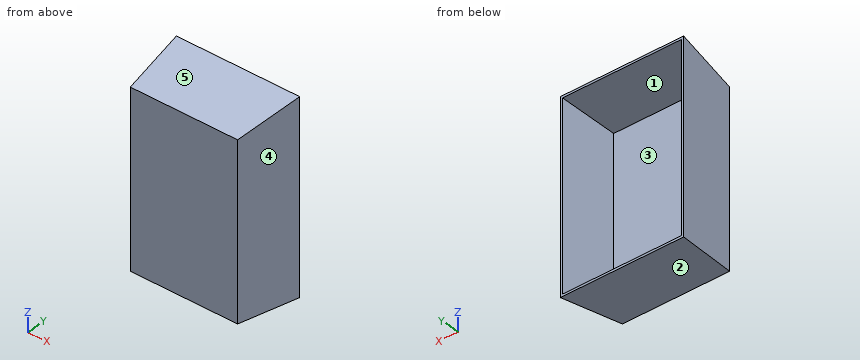
from build123d import *

# Parameters (mm, degrees)
SKETCH_1_W          = 475
SKETCH_1_H          = 780
EXTRUDE_1_DEPTH     = 289
EXTRUDE_1_DRAFT     = -7
SKETCH_2_W          = 525.969476202
SKETCH_2_H          = 830.969476202
CUT_EXTRUDE_1_DEPTH = 238
CUT_EXTRUDE_1_DRAFT = -7


with BuildPart() as part:
    # Эскиз1 → Бобышка-Вытянуть1 (with draft: the straight prism first)
    with BuildSketch(Plane(origin=(0, 0, 0), x_dir=(1, 0, 0), z_dir=(0, 1, 0))):
        with Locations((-465.395753162, -95.652339489)):
            Rectangle(SKETCH_1_W, SKETCH_1_H)
    extrude(amount=EXTRUDE_1_DEPTH)
    # Бобышка-Вытянуть1: the draft: its side faces are tilted about the plane it starts from
    extrude_1_sides = [part.faces().sort_by_distance(p)[0] for p in [
        (-465.395753162, 144.5, -294.347660511),
        (-702.895753162, 144.5, 95.652339489),
        (-465.395753162, 144.5, 485.652339489),
        (-227.895753162, 144.5, 95.652339489),
    ]]
    draft(extrude_1_sides, Plane(origin=(0, 0, 0), x_dir=(1, 0, 0), z_dir=(0, 1, 0)), EXTRUDE_1_DRAFT)


with BuildPart() as cut_extrude_1_tool:
    # Эскиз2 → Вырез-Вытянуть1 (with draft: the straight prism first)
    with BuildSketch(Plane(origin=(0, 289, 0), x_dir=(1, 0, 0), z_dir=(0, 1, 0))):
        with Locations((-465.395753162, -95.652339489)):
            Rectangle(SKETCH_2_W, SKETCH_2_H)
    extrude(amount=-CUT_EXTRUDE_1_DEPTH)
    # Вырез-Вытянуть1: the draft: its side faces are tilted about the plane it starts from
    cut_extrude_1_sides = [cut_extrude_1_tool.faces().sort_by_distance(p)[0] for p in [
        (-728.380491263, 170, 95.652339489),
        (-465.395753162, 170, 511.13707759),
        (-202.411015061, 170, 95.652339489),
        (-465.395753162, 170, -319.832398612),
    ]]
    draft(cut_extrude_1_sides, Plane(origin=(0, 289, 0), x_dir=(1, 0, 0), z_dir=(0, 1, 0)), CUT_EXTRUDE_1_DRAFT)


with BuildPart() as part_1:
    add(part.part)

    # Вырез-Вытянуть1: cut by cut_extrude_1_tool
    add(cut_extrude_1_tool.part, mode=Mode.SUBTRACT)


solid = part_1.part
Input: part model. Units: mm. Frame: model coordinates. Face numbers are marked on the shaded views. A direction names the side the tool comes from. Coordinates: 2 decimals unless noted, no trailing zeros. Order: outer loops, then holes, each group sorted by start corner. A loop starts at its lowest first (then second) coordinate and runs counter-clockwise, first axis right, second up. Notation, with made-up numbers: M 14,15.25 L 68,15.25 A33 cw 68,47.25 Z; hole C -30,80.5 d4. An arc over 180 degrees is marked long. Write item = value, one per line. Start each with the question number.
(1) First-contact query: P1, Ø1, axis at y = 181, z = 392, coming from the +X side; P2, Ø4, axis at y = 176.5, z = 99.5, coming from the -X side; P3, Ø12, axis at x = -497.5, y = 226, coming from the +Z side. Flat tips, straight axial feed; report the tip coordinate or a pass-through.
(2) Section B-B on y = 203. Output: boundary loops of the cut face in (x, z), and give its area (3 significant figures).
(3) Section C-C on x = -458. Output: boundary loops of the cut face in (y, z), and give its area (3 significant figures).
(4) Line query: line 1 along Y through (x, z) = (-494, 320); line 2 along X through (y, z) = (188, 234); line 3 along Z through (x, y) = (-405.5, 177). Output: solid intervals per line, ascending. Write a range as [from, to].
(5) Reachability of the marked faces 1 and 2 from +Z, -Z, +X, -X, +Y, -Y: full face, straight path, thin tool, end or side. Return the list, or none.
(6) Pull-direction query (X, two-part tool) for the marked faces 3, 4 and 5; classes: released by +X, released by -X, zero draft, split by the parting line, or undercut.
(7) Section D-D on y = 34. Output: boundary loops of the cut face in (x, z).
(8) Section A-A on z = 310. Output: boundary loops of the cut face in (x, y).
Result set:
q1.P1 = -205.61
q1.P2 = -724.81
q1.P3 = 514.14
q2.outline = M -727.82,-319.27 L -202.97,-319.27 L -202.97,510.58 L -727.82,510.58 Z; hole M -717.82,-309.27 L -212.97,-309.27 L -212.97,500.58 L -717.82,500.58 Z
q2.area = 26,700 mm²
q3.outline = M 0,-294.35 L 289,-329.83 L 289,-319.83 L 51,-290.61 L 51,481.91 L 289,511.14 L 289,521.14 L 0,485.65 Z
q3.area = 44,900 mm²
q4.line_1 = [0, 51]
q4.line_2 = [-725.98, -715.98], [-214.81, -204.81]
q4.line_3 = [-316.08, -306.08], [497.39, 507.39]
q5.face_1 = +Y
q5.face_2 = -Z, +X, -X, -Y
q6.face_3 = undercut
q6.face_4 = released by +X
q6.face_5 = zero draft
q7.outline = M -707.07,-298.52 L -223.72,-298.52 L -223.72,489.83 L -707.07,489.83 Z
q8.outline = M -738.38,289 L -702.9,0 L -227.9,0 L -192.41,289 L -202.41,289 L -231.63,51 L -699.16,51 L -728.38,289 Z
